Here's how the part is built. I have some questions about the finished solid (model axes, mm). Face numbers are marked on the shaded views. Round coordinates to 2 decimals unless told otherwise and drop trailing zeros. Order: outer loops, then holes, each group sorted by start corner. A loop starts at its lowest first (then second) coordinate and runs counter-clockwise, first axis right, second up. Notation, with made-up numbers: (36.5, -4) -> (69.5, -4) arc R24 ccw to (69.5, 7) -> close; hole circle Ø11 at (28, 84). An arc over 180 degrees is marked (long way). Answer in a Markdown table with one row per item.
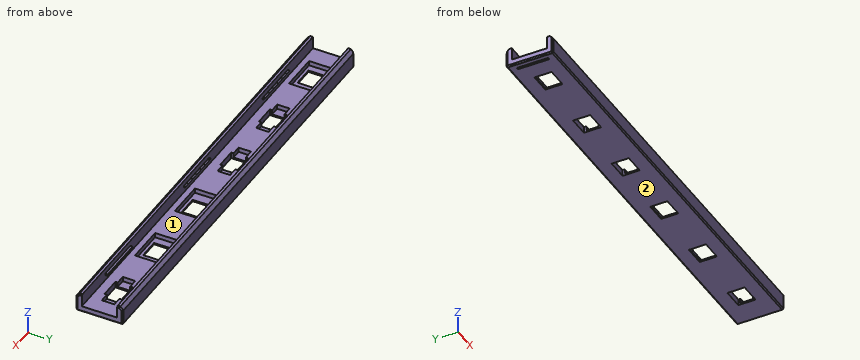
```python
from build123d import *

# Parameters (mm, degrees)
SKETCH1_W               = 138
SKETCH1_H               = 15
BOSS_EXTRUDE1_DEPTH     = 6
CUT_EXTRUDE1_DEPTH      = 96.457872636
CUT_EXTRUDE1_DEPTH_BACK = 96.457872636
SKETCH2_W               = 6.5
SKETCH2_H               = 5.5
CUT_EXTRUDE2_DEPTH      = 96.457872636
CUT_EXTRUDE2_DEPTH_BACK = 96.457872636
SKETCH3_W               = 6.5
SKETCH3_H               = 5.5
CUT_EXTRUDE3_DEPTH      = 96.457872636
CUT_EXTRUDE3_DEPTH_BACK = 96.457872636
SKETCH4_W               = 6.5
SKETCH4_H               = 5.5
CUT_EXTRUDE4_DEPTH      = 96.457872636
CUT_EXTRUDE4_DEPTH_BACK = 96.457872636
SKETCH5_W               = 6.5
SKETCH5_H               = 5.5
CUT_EXTRUDE5_DEPTH      = 96.457872636
CUT_EXTRUDE5_DEPTH_BACK = 4
SKETCH8_W               = 138
SKETCH8_H               = 11.3
SKETCH9_W               = 12
SKETCH9_H               = 7.5
SKETCH9_W_2             = 12.5
SKETCH9_H_2             = 4
CUT_EXTRUDE6_DEPTH      = 1.5
SKETCH10_W              = 12.5
SKETCH10_H              = 4
CUT_EXTRUDE7_DEPTH      = 1.5
CUT_EXTRUDE8_DEPTH      = 138
SKETCH13_W              = 0.5
SKETCH13_H              = 10
CUT_EXTRUDE9_DEPTH      = 0.6
FILLET1_R               = 0.25
FILLET2_R               = 0.25
SKETCH16_W              = 15
SKETCH16_H              = 0.5
BOSS_EXTRUDE2_DEPTH     = 0.75
FILLET3_R               = 0.5
FILLET4_R               = 0.25
SKETCH17_W              = 15
SKETCH17_H              = 0.5
BOSS_EXTRUDE3_DEPTH     = 0.75
FILLET5_R               = 0.5
FILLET6_R               = 0.25
LPATTERN1_COUNT         = 3
LPATTERN1_PITCH         = 47
LPATTERN2_COUNT         = 3
LPATTERN2_PITCH         = 47
FILLET7_R               = 0.5
FILLET8_R               = 0.25
FILLET9_R               = 0.5
FILLET10_R              = 0.25
CHAMFER1_SIZE           = 0.4
CHAMFER2_SIZE           = 0.4
CHAMFER3_SIZE           = 0.4
CHAMFER5_SIZE           = 0.4


# Some blends are built 0.0001 mm under size
with BuildPart() as part:
    # Sketch1 → Boss-Extrude1 (new body)
    with BuildSketch(Plane.XY):
        with Locations((-22.75, 18.154296875)):
            Rectangle(SKETCH1_W, SKETCH1_H)
    extrude(amount=BOSS_EXTRUDE1_DEPTH)

    # Sketch2 → Cut-Extrude1 (cut, two sides: drawn at the far end of the back side and taken through both)
    with BuildSketch(Plane.XY.offset(6).offset(-CUT_EXTRUDE1_DEPTH_BACK)):
        with Locations((-80.4, 18.154296875)):
            Rectangle(SKETCH2_W, SKETCH2_H)
    extrude(amount=CUT_EXTRUDE1_DEPTH + CUT_EXTRUDE1_DEPTH_BACK, mode=Mode.SUBTRACT)

    # Sketch3 → Cut-Extrude2 (cut, two sides: drawn at the far end of the back side and taken through both)
    with BuildSketch(Plane.XY.offset(6).offset(-CUT_EXTRUDE2_DEPTH_BACK)):
        with Locations((-57.35, 18.154296875)):
            Rectangle(SKETCH3_W, SKETCH3_H)
    extrude(amount=CUT_EXTRUDE2_DEPTH + CUT_EXTRUDE2_DEPTH_BACK, mode=Mode.SUBTRACT)

    # Sketch4 → Cut-Extrude3 (cut, two sides: drawn at the far end of the back side and taken through both)
    with BuildSketch(Plane.XY.offset(6).offset(-CUT_EXTRUDE3_DEPTH_BACK)):
        with Locations((-34.3, 18.154296875)):
            Rectangle(SKETCH4_W, SKETCH4_H)
    extrude(amount=CUT_EXTRUDE3_DEPTH + CUT_EXTRUDE3_DEPTH_BACK, mode=Mode.SUBTRACT)

    # Sketch5 → Cut-Extrude4 (cut, two sides: drawn at the far end of the back side and taken through both)
    with BuildSketch(Plane.XY.offset(6).offset(-CUT_EXTRUDE4_DEPTH_BACK)):
        with Locations((-11.25, 18.154296875)):
            Rectangle(SKETCH5_W, SKETCH5_H)
        with Locations((11.8, 18.154296875)):
            Rectangle(SKETCH5_W, SKETCH5_H)
        with Locations((34.85, 18.154296875)):
            Rectangle(SKETCH5_W, SKETCH5_H)
    extrude(amount=CUT_EXTRUDE4_DEPTH + CUT_EXTRUDE4_DEPTH_BACK, mode=Mode.SUBTRACT)

    # Sketch8 → Cut-Extrude5 (cut, two sides: drawn at the far end of the back side and taken through both)
    with BuildSketch(Plane.XY.offset(6).offset(-CUT_EXTRUDE5_DEPTH_BACK)):
        with Locations((-22.75, 18.154296875)):
            Rectangle(SKETCH8_W, SKETCH8_H)
    extrude(amount=CUT_EXTRUDE5_DEPTH + CUT_EXTRUDE5_DEPTH_BACK, mode=Mode.SUBTRACT)

    # Sketch9 → Cut-Extrude6 (cut)
    with BuildSketch(Plane.XY.offset(2)):
        with Locations((-11.75, 18.154296875)):
            Rectangle(SKETCH9_W, SKETCH9_H)
        with Locations((12.05, 18.154296875)):
            Rectangle(SKETCH9_W, SKETCH9_H)
        with Locations((-79.9, 18.154296875)):
            Rectangle(SKETCH9_W, SKETCH9_H)
        with Locations((34.85, 18.154296875)):
            Rectangle(SKETCH9_W_2, SKETCH9_H_2)
    extrude(amount=-CUT_EXTRUDE6_DEPTH, mode=Mode.SUBTRACT)

    # Sketch10 → Cut-Extrude7 (cut)
    with BuildSketch(Plane.XY.offset(2)):
        with Locations((-34.3, 18.154296875)):
            Rectangle(SKETCH10_W, SKETCH10_H)
        with Locations((-57.35, 18.154296875)):
            Rectangle(SKETCH10_W, SKETCH10_H)
    extrude(amount=-CUT_EXTRUDE7_DEPTH, mode=Mode.SUBTRACT)

    # Sketch12 → Cut-Extrude8 (cut)
    with BuildSketch(Plane(origin=(46.25, 0, 0), x_dir=(0, 0, -1), z_dir=(1, 0, 0))):
        Polygon((-6, 25.654296875), (-6, 24.654296875), (-5, 25.654296875), align=None)
        Polygon((-6, 10.654296875), (-5, 10.654296875), (-6, 11.654296875), align=None)
    extrude(amount=-CUT_EXTRUDE8_DEPTH, mode=Mode.SUBTRACT)

    # Sketch13 → Cut-Extrude9 (cut)
    with BuildSketch(Plane(origin=(0, 0, 0), x_dir=(-1, 0, 0), z_dir=(0, 0, -1))):
        with Locations((89.5, 18.154296875)):
            Rectangle(SKETCH13_W, SKETCH13_H)
    extrude(amount=-CUT_EXTRUDE9_DEPTH, mode=Mode.SUBTRACT)

    # Fillet1
    fillet1_edges = [part.edges().sort_by_distance(p)[0] for p in [
        (-89.75, 18.154296875, 0),
    ]]
    fillet(fillet1_edges, radius=FILLET1_R)

    # Fillet2
    fillet2_edges = [part.edges().sort_by_distance(p)[0] for p in [
        (-89.25, 18.154296875, 0.6),
        (-89.5, 23.154296875, 0.6),
        (-89.75, 18.154296875, 0.6),
        (-89.5, 13.154296875, 0.6),
    ]]
    fillet(fillet2_edges, radius=FILLET2_R - 0.0001)  # a hair under: the kernel refuses the full size

    # Sketch16 → Boss-Extrude2 (add)
    with BuildSketch(Plane.XZ.offset(-23.804296875)):
        with Locations((-69.25, 4)):
            Rectangle(SKETCH16_W, SKETCH16_H)
    boss_extrude2 = extrude(amount=BOSS_EXTRUDE2_DEPTH)

    # Fillet3
    fillet3_edges = [part.edges().sort_by_distance(p)[0] for p in [
        (-69.25, 23.054296875, 4.25),
    ]]
    fillet(fillet3_edges, radius=FILLET3_R - 0.0001)  # a hair under: the kernel refuses the full size

    # Fillet4
    # the kernel refuses this fillet: 0.25 mm, written as the material it takes off along each edge
    with BuildSketch(Plane(origin=(-78.517583771, 23.054296875, 3.75), x_dir=(0, 0.7070334963750315, 0.7071800584035852), z_dir=(1, 0, 0))) as fillet4_piece_1:
        with BuildLine():
            CenterArc((0.530239778, -0.176759656), FILLET4_R, 44.994477546, 179.999584605)
            Line((0.353444764, -0.35351803), (0.335765262, -0.371193867))
            Line((0.335765262, -0.371193867), (-0.017679501, -0.017675837))
            Line((-0.017679501, -0.017675837), (-0.017675837, 0.017679501))
            ThreePointArc((-0.017675837, 0.017679501), (-0.017605119, 0.017750205), (0.724712885, 0.017675966))
            Line((0.724712885, 0.017675966), (0.707033512, 0))
        make_face()
    extrude(amount=18.535167542, mode=Mode.SUBTRACT)

    # Sketch17 → Boss-Extrude3 (add)
    with BuildSketch(Plane(origin=(0, 12.504296875, 0), x_dir=(1, 0, 0), z_dir=(0, 1, 0))):
        with Locations((-69.25, -4)):
            Rectangle(SKETCH17_W, SKETCH17_H)
    boss_extrude3 = extrude(amount=BOSS_EXTRUDE3_DEPTH)

    # Fillet5
    fillet5_edges = [part.edges().sort_by_distance(p)[0] for p in [
        (-69.25, 13.254296875, 4.25),
    ]]
    fillet(fillet5_edges, radius=FILLET5_R - 0.0001)  # a hair under: the kernel refuses the full size

    # Fillet6
    # the kernel refuses this fillet: 0.25 mm, written as the material it takes off along each edge
    with BuildSketch(Plane(origin=(-59.982416237, 13.254296875, 3.75), x_dir=(0, -0.707033490014658, 0.7071800647626406), z_dir=(-1, 0, 0))) as fillet6_piece_1:
        with BuildLine():
            CenterArc((0.530239774, -0.176759657), FILLET6_R, 44.994478062, 179.999583575)
            Line((0.353444757, -0.35351803), (0.335765256, -0.371193867))
            Line((0.335765256, -0.371193867), (-0.017679502, -0.017675837))
            Line((-0.017679502, -0.017675837), (-0.017675837, 0.017679502))
            ThreePointArc((-0.017675837, 0.017679502), (-0.017605119, 0.017750205), (0.724712878, 0.017675966))
            Line((0.724712878, 0.017675966), (0.707033505, 0))
        make_face()
    extrude(amount=18.535167526, mode=Mode.SUBTRACT)

    # LPattern1: Boss-Extrude3 ×3
    with Locations(*[(i * LPATTERN1_PITCH, 0, 0) for i in range(1, LPATTERN1_COUNT)]):
        add(boss_extrude3)

    # LPattern2: Boss-Extrude2 ×3
    with Locations(*[(i * LPATTERN2_PITCH, 0, 0) for i in range(1, LPATTERN2_COUNT)]):
        add(boss_extrude2)

    # Fillet7
    fillet7_edges = [part.edges().sort_by_distance(p)[0] for p in [
        (-22.25, 23.054296875, 4.25),
    ]]
    fillet(fillet7_edges, radius=FILLET7_R - 0.0001)  # a hair under: the kernel refuses the full size

    # Fillet8
    # the kernel refuses this fillet: 0.25 mm, written as the material it takes off along each edge
    with BuildSketch(Plane(origin=(-31.517583771, 23.054296875, 3.75), x_dir=(0, 0.7070334900866685, 0.707180064690645), z_dir=(1, 0, 0))) as fillet8_piece_1:
        with BuildLine():
            CenterArc((0.530239774, -0.176759657), FILLET8_R, 44.994478056, 179.999583586)
            Line((0.353444758, -0.35351803), (0.335765256, -0.371193867))
            Line((0.335765256, -0.371193867), (-0.017679502, -0.017675837))
            Line((-0.017679502, -0.017675837), (-0.017675837, 0.017679502))
            ThreePointArc((-0.017675837, 0.017679502), (-0.017605119, 0.017750205), (0.724712878, 0.017675966))
            Line((0.724712878, 0.017675966), (0.707033505, 0))
        make_face()
    extrude(amount=18.535167542, mode=Mode.SUBTRACT)

    # Fillet9
    fillet9_edges = [part.edges().sort_by_distance(p)[0] for p in [
        (-22.25, 13.254296875, 4.25),
    ]]
    fillet(fillet9_edges, radius=FILLET9_R - 0.0001)  # a hair under: the kernel refuses the full size

    # Fillet10
    # the kernel refuses this fillet: 0.25 mm, written as the material it takes off along each edge
    with BuildSketch(Plane(origin=(-12.982416233, 13.254296875, 3.75), x_dir=(0, -0.7070334900159922, 0.7071800647613065), z_dir=(-1, 0, 0))) as fillet10_piece_1:
        with BuildLine():
            CenterArc((0.530239774, -0.176759657), FILLET10_R, 44.994478062, 179.999583575)
            Line((0.353444757, -0.35351803), (0.335765256, -0.371193867))
            Line((0.335765256, -0.371193867), (-0.017679502, -0.017675837))
            Line((-0.017679502, -0.017675837), (-0.017675837, 0.017679502))
            ThreePointArc((-0.017675837, 0.017679502), (-0.017605119, 0.017750205), (0.724712878, 0.017675966))
            Line((0.724712878, 0.017675966), (0.707033505, 0))
        make_face()
    extrude(amount=18.535167534, mode=Mode.SUBTRACT)

    # Chamfer1
    chamfer1_edges = [part.edges().sort_by_distance(p)[0] for p in [
        (-22.75, 25.654296875, 0),
        (-22.75, 10.654296875, 0),
    ]]
    chamfer(chamfer1_edges, length=CHAMFER1_SIZE)

    # Chamfer2
    chamfer2_edges = [part.edges().sort_by_distance(p)[0] for p in [
        (46.25, 18.154296875, 0),
        (-91.75, 18.154296875, 0),
    ]]
    chamfer(chamfer2_edges, length=CHAMFER2_SIZE)

    # Chamfer3
    chamfer3_edges = [part.edges().sort_by_distance(p)[0] for p in [
        (-91.75, 25.654296875, 2.7),
        (-91.75, 10.654296875, 2.7),
    ]]
    chamfer(chamfer3_edges, length=CHAMFER3_SIZE)

    # Chamfer5
    chamfer5_edges = [part.edges().sort_by_distance(p)[0] for p in [
        (46.25, 24.229296875, 6),
        (46.25, 25.654296875, 2.7),
        (46.25, 10.654296875, 2.7),
        (46.25, 12.079296875, 6),
        (46.25, 25.154296875, 5.5),
        (46.25, 11.154296875, 5.5),
    ]]
    chamfer(chamfer5_edges, length=CHAMFER5_SIZE)


solid = part.part
```
1. For pin 1 Ø5 at (x, y) = (-37, 19.5) entering from +Z, with a flat end and sliding along its axis, tell me the tip position at first contact or that it passes through.
Numbers:
| item | result |
|---|---|
| pin 1 | stops at z = 2 |
2. We'd pull the mould along Y, two halves only. Please class the marked faces 1 and 2: released by +Y, released by -Y, zero draft, split by the parting line, or undercut.
Numbers:
| item | result |
|---|---|
| face 1 | undercut |
| face 2 | zero draft |
3. Suppose I cut it at A-A on x = -82.5. Write out the boundary of the cut face in (y, z).
Numbers:
| item | result |
|---|---|
| outline | (10.65, 0.4) -> (11.05, 0) -> (15.4, 0) -> (15.4, 0.5) -> (14.4, 0.5) -> (14.4, 2) -> (12.5, 2) -> (12.5, 6) -> (11.65, 6) -> (10.65, 5) -> close; (20.9, 0) -> (25.25, 0) -> (25.65, 0.4) -> (25.65, 5) -> (24.65, 6) -> (23.8, 6) -> (23.8, 2) -> (21.9, 2) -> (21.9, 0.5) -> (20.9, 0.5) -> close |
4. Please list where these lines run through material, in increasing order: line 1 along Y through (x, z) = (-32.5, 2.25); line 2 along X through (y, z) = (15, 1.5); line 3 along Y through (x, z) = (-8.5, 1.75).
Numbers:
| item | result |
|---|---|
| line 1 | y = 10.65 to 12.5, 23.8 to 25.65 |
| line 2 | x = -91.75 to -85.9, -73.9 to -17.75, -5.75 to 6.05, 18.05 to 46.25 |
| line 3 | y = 10.65 to 14.4, 21.9 to 25.65 |
5. Suppose I cut it at B-B on x = -43. Write out the boundary of the cut face in (y, z), then the cut area to 3 significant figures.
Numbers:
| item | result |
|---|---|
| outline | (10.65, 0.4) -> (11.05, 0) -> (25.25, 0) -> (25.65, 0.4) -> (25.65, 5) -> (24.65, 6) -> (23.8, 6) -> (23.8, 2) -> (12.5, 2) -> (12.5, 6) -> (11.65, 6) -> (10.65, 5) -> close |
| area | 43.6 mm2 |
